Study the drawing (mm; zero at the part's minimum x, y, z) and answer. Give positions to 0.01 mm unless a question says otherwise; leave off trailing zeros. Write each loop counter-clockwise with the first axis right and the second up, starting at its lowest first coordinate (ties: lowest second). Pieces come first, ordered by that corner, then holes.
1) Determine the mould class of the marked faces 1, 2, 3 and 4 for opening direction X: pulls with the +X half, pulls with the -X half, needs draft (parallel to the pull), parting line crosses it, or undercut.
2) Find section D-D (y = 21). Determine the outline of the cut face in (x, z).
3) Given pin 1 Ø7 at (x, z) = (28, 16) entering from -Y; pin 2 Ø5 at (y, z) = (9, 145.5) entering from -X; pin 3 Ø6 at (x, y) = (45, 16.5) entering from +Z; pin 4 Ø14 at (x, z) = (28, 159) entering from +Y, each flat-ended and moving along its own axis, determine where each tip first touches the part or whether it passes through.
4) Find section C-C (x = 6.5). Determine the outline of the cut face in (y, z).
5) Straight lines are drawn through the part: probe 1 along X at (y, z) = (4, 16); probe 2 along X at (y, z) = (19, 44.5); probe 3 along Z at (x, y) = (23.5, 4.5). For each, find the intervals that lie inside material, in ascending order.
6) Find section A-A (z = 16). Determine the outline of the cut face in (x, y), plus the area to 3 significant figures.
7) Find section B-B (x = 28). Determine the outline of the cut face in (y, z), plus the area to 3 significant figures.
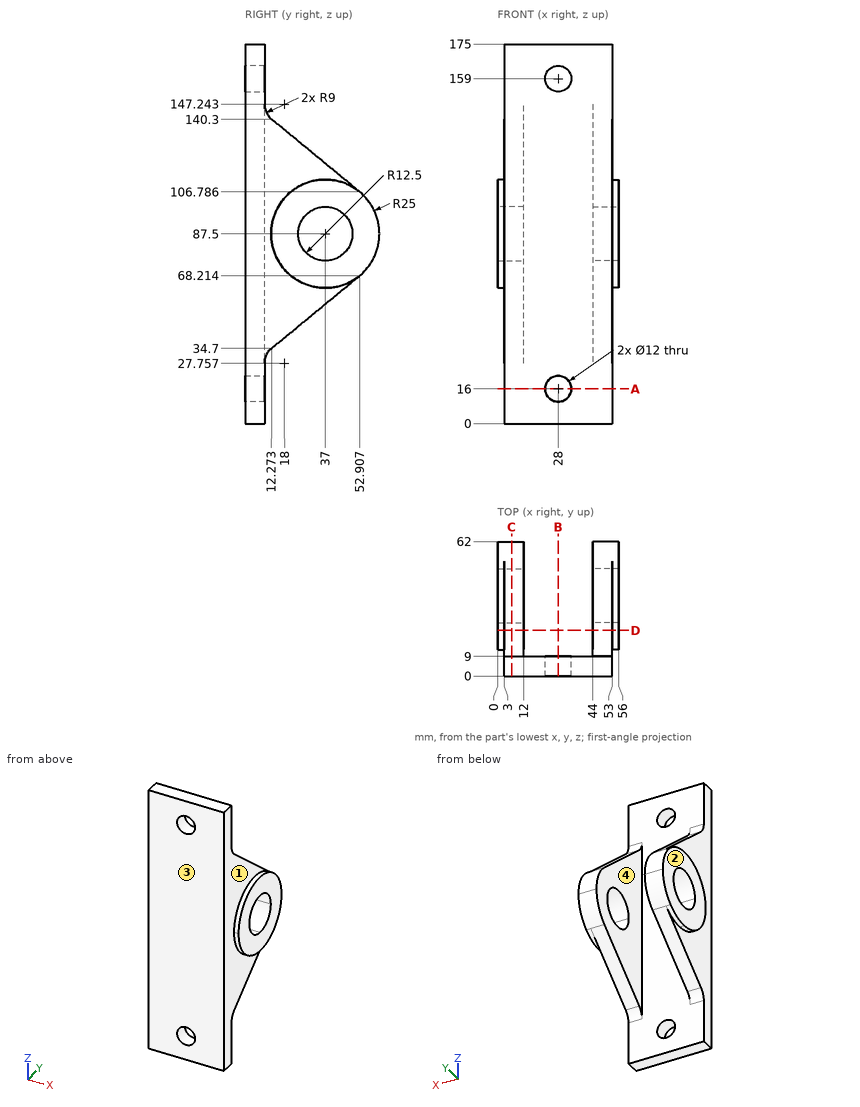
Results:
1. face 1: pulls with the +X half
1. face 2: pulls with the -X half
1. face 3: needs draft
1. face 4: undercut
2. outline: (0, 68.29) - (3, 68.29) - (3, 41.9) - (12, 41.9) - (12, 133.1) - (3, 133.1) - (3, 106.71) - (0, 106.71) - close; (44, 41.9) - (53, 41.9) - (53, 68.29) - (56, 68.29) - (56, 106.71) - (53, 106.71) - (53, 133.1) - (44, 133.1) - close
3. pin 1: passes through
3. pin 2: stops at x = 3
3. pin 3: stops at z = 139.29
3. pin 4: stops at y = 9
4. outline: (0, 0) - (9, 0) - (9, 27.76) arc R9 cw to (12.27, 34.7) - (52.91, 68.21) arc R25 ccw to (52.91, 106.79) - (12.27, 140.3) arc R9 cw to (9, 147.24) - (9, 175) - (0, 175) - close; hole circle Ø25 at (37, 87.5)
5. probe 1: x = 3 to 22, 34 to 53
5. probe 2: x = 3 to 12, 44 to 53
5. probe 3: z = 0 to 12.03, 19.97 to 155.03, 162.97 to 175
6. outline: (3, 0) - (22, 0) - (22, 9) - (3, 9) - close; (34, 0) - (53, 0) - (53, 9) - (34, 9) - close
6. area: 342 mm2
7. outline: (0, 0) - (9, 0) - (9, 10) - (0, 10) - close; (0, 22) - (9, 22) - (9, 153) - (0, 153) - close; (0, 165) - (9, 165) - (9, 175) - (0, 175) - close
7. area: 1,360 mm2
